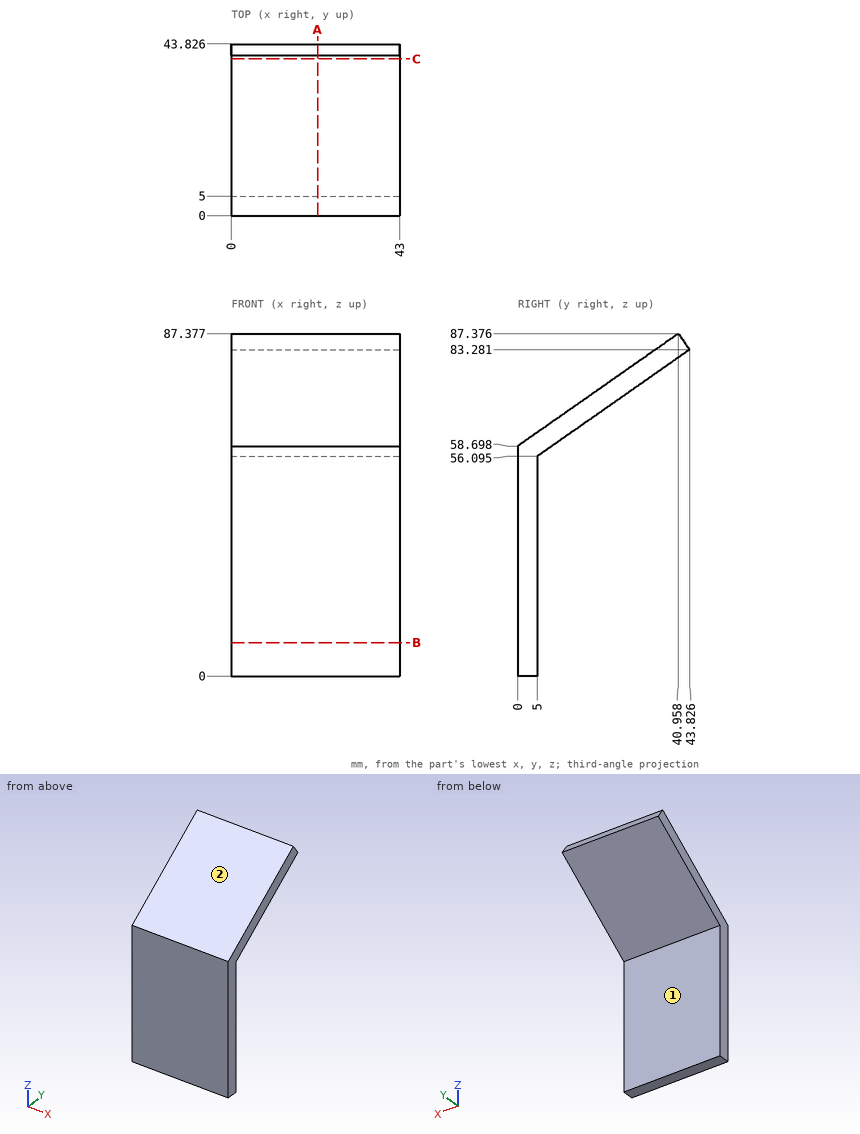
Study the drawing (mm; zero at the part's minimum x, y, z) and answer. A direction names the side the tool comes from. Give positions to 0.01 mm unless a question says otherwise; leave off trailing zeros. Order: outer loops, then holes, each group sorted by start corner. A loop starts at its lowest first (then second) coordinate and runs counter-clockwise, first axis right, second up. Notation, with made-up numbers: (-31.75, 22.25) - (13.25, 22.25) arc R24 cw to (13.25, 54.25) - close; hole circle Ø5 at (42.5, 51.25). An arc over 180 degrees is marked (long way). Answer in a Markdown table with one row per item. Add a question column.
Q1. The part is cut by section A-A (x = 22). Determine the outline of the cut face in (y, z) (1 decimal).
Q2. Find the intervals of material crossed by line 1 along Y through (x, z) = (20, 53); line 2 along Z through (x, y) = (12.5, 25) (1 decimal); line 3 along Z through (x, y) = (29, 23.5), in increasing order. Write a range as [from, to].
Q3. Which of the six approach directions +Z, -Z, +X, -X, +Y, -Y give full straight-line access (tool end or side, diameter ignored) to the marked faces 1 and 2?
Q4. The part is cut by section B-B (z = 8.5). Determine the outline of the cut face in (x, y), then the cut area to 3 significant figures.
Q5. The part is cut by section C-C (y = 40). Determine the outline of the cut face in (x, z) (1 decimal).
Q6. Given P1, Ø6, axis at x = 33, z = 37, coming from the +Y side; P2, Ø1.5, axis at y = 22.5, z = 75.5, coming from the +X side; P3, Ø12, axis at x = 18, z = 55.5, coming from the +Y side; P4, Ø8, axis at x = 8, z = 73.5, coming from the +Y side, each flat-ended and moving along its own axis, determine where each tip first touches the part or whether it passes through.
Determined:
| question | item | result |
|---|---|---|
| 1 | outline | (0, 0) - (5, 0) - (5, 56.1) - (43.8, 83.3) - (41, 87.4) - (0, 58.7) - close |
| 2 | line 1 | y = [0, 5] |
| 2 | line 2 | z = [70.1, 76.2] |
| 2 | line 3 | z = [69.05, 75.15] |
| 3 | face 1 | -Z, +X, -X, +Y |
| 3 | face 2 | +Z, +X, -X, -Y |
| 4 | outline | (0, 0) - (43, 0) - (43, 5) - (0, 5) - close |
| 4 | area | 215 mm² |
| 5 | outline | (0, 80.6) - (43, 80.6) - (43, 86.7) - (0, 86.7) - close |
| 6 | P1 | stops at y = 5 |
| 6 | P2 | passes through |
| 6 | P3 | stops at y = 12.72 |
| 6 | P4 | stops at y = 35.57 |
